Work out the finished part from the listing and answer in its coordinate system (mm). Round coordinates to 2 decimals unless told otherwise and drop trailing zeros. Loops run counter-clockwise (first coordinate to the right, second up) from the corner with the lowest first, then second, coordinate; pieces in that order, holes last.
```python
from build123d import *

# Parameters (mm, degrees)
SKETCH1_R                                         = 82.55
BASE_DEPTH                                        = 6.35
CSK_FOR_6_FLAT_HEAD_MACHINE_SCREW_100_D           = 3.7973
CSK_FOR_6_FLAT_HEAD_MACHINE_SCREW_100_CSINK_D     = 7.0866
CSK_FOR_6_FLAT_HEAD_MACHINE_SCREW_100_CSINK_ANGLE = 100
CUT_EXTRUDE1_DEPTH                                = 117.915899261
F_10_0_1935_DIAMETER_HOLE1_AT_2_COUNT             = 2
F_10_0_1935_DIAMETER_HOLE1_AT_2_PITCH             = 19.05
F_10_0_1935_DIAMETER_HOLE1_AT_3_COUNT             = 2
F_10_0_1935_DIAMETER_HOLE1_AT_3_PITCH             = 25.208780216
F_10_0_1935_DIAMETER_HOLE1_AT_4_COUNT             = 2
F_10_0_1935_DIAMETER_HOLE1_AT_4_PITCH             = 16.51
CIRPATTERN1_COUNT                                 = 3
CUT_EXTRUDE3_DEPTH                                = 117.915899261
FILLET1_R                                         = 7.62
F_8_0_199_DIAMETER_HOLE1_D                        = 5.0546


with BuildPart() as part:
    # Sketch1 → Base (new body)
    with BuildSketch(Plane.XY):
        Circle(SKETCH1_R)
    extrude(amount=BASE_DEPTH)

    # CSK for _6 Flat Head Machine Screw _100 (through all)
    with Locations(Plane(origin=(0, 0, 0), x_dir=(-1, 0, 0), z_dir=(0, 0, -1))):
        with Locations((-41.5, 9), (-41.5, -9), (42.95, 9), (42.95, -9)):
            CounterSinkHole(CSK_FOR_6_FLAT_HEAD_MACHINE_SCREW_100_D / 2, CSK_FOR_6_FLAT_HEAD_MACHINE_SCREW_100_CSINK_D / 2, counter_sink_angle=CSK_FOR_6_FLAT_HEAD_MACHINE_SCREW_100_CSINK_ANGLE)

    # Sketch8 → Cut-Extrude1 (cut, through all)
    with BuildSketch(Plane(origin=(0, 0, 0), x_dir=(-1, 0, 0), z_dir=(0, 0, -1))):
        with BuildLine():
            Line((40, -72.21151224), (-40, -72.21151224))
            ThreePointArc((-40, -72.21151224), (0, -82.55), (40, -72.21151224))
        make_face()
    extrude(amount=-CUT_EXTRUDE1_DEPTH, mode=Mode.SUBTRACT)

    # Sketch12 → #10 (0.1935) Diameter Hole1 (revolve, cut)
    with BuildSketch(Plane(origin=(-40.881368906, -34.601391971, 0), x_dir=(0, 1, 0), z_dir=(1, 0, 0))):
        Polygon((0, 0), (0, 7.826584928), (2.45745, 6.35), (2.45745, 0), align=None)
    f_10_0_1935_diameter_hole1 = revolve(axis=Axis((-40.881368906, -34.601391971, -6.35), (0, 0, 1)), mode=Mode.SUBTRACT)

    # #10 (0.1935) Diameter Hole1 at 2: #10 (0.1935) Diameter Hole1 ×2
    with Locations(*[Vector(-0.4999999999999995, 0.866025403784439, 0) * (i * F_10_0_1935_DIAMETER_HOLE1_AT_2_PITCH) for i in range(1, F_10_0_1935_DIAMETER_HOLE1_AT_2_COUNT)]):
        add(f_10_0_1935_diameter_hole1, mode=Mode.SUBTRACT)

    # #10 (0.1935) Diameter Hole1 at 3: #10 (0.1935) Diameter Hole1 ×2
    with Locations(*[Vector(-0.9450310253789799, 0.32698067384962365, 0) * (i * F_10_0_1935_DIAMETER_HOLE1_AT_3_PITCH) for i in range(1, F_10_0_1935_DIAMETER_HOLE1_AT_3_COUNT)]):
        add(f_10_0_1935_diameter_hole1, mode=Mode.SUBTRACT)

    # #10 (0.1935) Diameter Hole1 at 4: #10 (0.1935) Diameter Hole1 ×2
    with Locations(*[Vector(-0.8660254037844388, -0.49999999999999967, 0) * (i * F_10_0_1935_DIAMETER_HOLE1_AT_4_PITCH) for i in range(1, F_10_0_1935_DIAMETER_HOLE1_AT_4_COUNT)]):
        add(f_10_0_1935_diameter_hole1, mode=Mode.SUBTRACT)

    # CirPattern1: #10 (0.1935) Diameter Hole1 ×3 about axis
    cirpattern1_axis = Axis((0, 0, 0), (0, 0, 1))
    for i in range(1, CIRPATTERN1_COUNT):
        add(f_10_0_1935_diameter_hole1.rotate(cirpattern1_axis, i * 360 / CIRPATTERN1_COUNT), mode=Mode.SUBTRACT)

    # CirPattern1 copy 1 sketch → CirPattern1 copy 1 (revolve, cut)
    with BuildSketch(Plane(origin=(40.881368906, -34.601391971, 0), x_dir=(-0.8660254037844387, -0.4999999999999998, 0), z_dir=(-0.4999999999999998, 0.8660254037844387, 0))):
        Polygon((0, 0), (0, 7.826584928), (2.45745, 6.35), (2.45745, 0), align=None)
    revolve(axis=Axis((40.881368906, -34.601391971, -6.35), (0, 0, 1)), mode=Mode.SUBTRACT)

    # CirPattern1 copy 2 sketch → CirPattern1 copy 2 (revolve, cut)
    with BuildSketch(Plane(origin=(9.525, 52.705, 0), x_dir=(0.8660254037844384, -0.5000000000000004, 0), z_dir=(-0.5000000000000004, -0.8660254037844384, 0))):
        Polygon((0, 0), (0, 7.826584928), (2.45745, 6.35), (2.45745, 0), align=None)
    revolve(axis=Axis((9.525, 52.705, -6.35), (0, 0, 1)), mode=Mode.SUBTRACT)

    # CirPattern1 copy 3 sketch → CirPattern1 copy 3 (revolve, cut)
    with BuildSketch(Plane(origin=(55.179448323, -42.856391971, 0), x_dir=(-0.8660254037844387, -0.4999999999999998, 0), z_dir=(-0.4999999999999998, 0.8660254037844387, 0))):
        Polygon((0, 0), (0, 7.826584928), (2.45745, 6.35), (2.45745, 0), align=None)
    revolve(axis=Axis((55.179448323, -42.856391971, -6.35), (0, 0, 1)), mode=Mode.SUBTRACT)

    # CirPattern1 copy 4 sketch → CirPattern1 copy 4 (revolve, cut)
    with BuildSketch(Plane(origin=(9.525, 69.215, 0), x_dir=(0.8660254037844384, -0.5000000000000004, 0), z_dir=(-0.5000000000000004, -0.8660254037844384, 0))):
        Polygon((0, 0), (0, 7.826584928), (2.45745, 6.35), (2.45745, 0), align=None)
    revolve(axis=Axis((9.525, 69.215, -6.35), (0, 0, 1)), mode=Mode.SUBTRACT)

    # CirPattern1 copy 5 sketch → CirPattern1 copy 5 (revolve, cut)
    with BuildSketch(Plane(origin=(64.704448323, -26.358608029, 0), x_dir=(-0.8660254037844387, -0.4999999999999998, 0), z_dir=(-0.4999999999999998, 0.8660254037844387, 0))):
        Polygon((0, 0), (0, 7.826584928), (2.45745, 6.35), (2.45745, 0), align=None)
    revolve(axis=Axis((64.704448323, -26.358608029, -6.35), (0, 0, 1)), mode=Mode.SUBTRACT)

    # CirPattern1 copy 6 sketch → CirPattern1 copy 6 (revolve, cut)
    with BuildSketch(Plane(origin=(-9.525, 69.215, 0), x_dir=(0.8660254037844384, -0.5000000000000004, 0), z_dir=(-0.5000000000000004, -0.8660254037844384, 0))):
        Polygon((0, 0), (0, 7.826584928), (2.45745, 6.35), (2.45745, 0), align=None)
    revolve(axis=Axis((-9.525, 69.215, -6.35), (0, 0, 1)), mode=Mode.SUBTRACT)

    # Sketch14 → Cut-Extrude3 (cut, through all)
    with BuildSketch(Plane.XY.offset(6.35)):
        with BuildLine():
            Line((-28.575, 28.05), (-123.194399556, 28.05))
            Line((-123.194399556, 28.05), (-123.194399556, 124.921419199))
            Line((-123.194399556, 124.921419199), (-18.415, 124.921419199))
            Line((-18.415, 124.921419199), (-18.415, 38.21))
            ThreePointArc((-18.415, 38.21), (-21.390795103, 31.025795103), (-28.575, 28.05))
        make_face()
        with BuildLine():
            Line((123.194399556, 28.05), (123.194399556, 124.921419199))
            Line((123.194399556, 124.921419199), (18.415, 124.921419199))
            Line((18.415, 124.921419199), (18.415, 38.21))
            ThreePointArc((18.415, 38.21), (21.390795103, 31.025795103), (28.575, 28.05))
            Line((28.575, 28.05), (123.194399556, 28.05))
        make_face()
    extrude(amount=-CUT_EXTRUDE3_DEPTH, mode=Mode.SUBTRACT)

    # Fillet1
    fillet1_edges = [part.edges().sort_by_distance(p)[0] for p in [
        (-18.415, 80.469809711, 3.175),
        (-77.638263762, 28.05, 3.175),
        (18.415, 80.469809711, 3.175),
        (77.638263762, 28.05, 3.175),
    ]]
    fillet(fillet1_edges, radius=FILLET1_R)

    # #8 (0.199) Diameter Hole1 (through all)
    with Locations(Plane(origin=(0, 0, 0), x_dir=(-1, 0, 0), z_dir=(0, 0, -1))):
        with Locations((47.715, -48.08151224), (0.725, -48.08151224), (-46.265, -48.08151224)):
            Hole(F_8_0_199_DIAMETER_HOLE1_D / 2)


solid = part.part
```
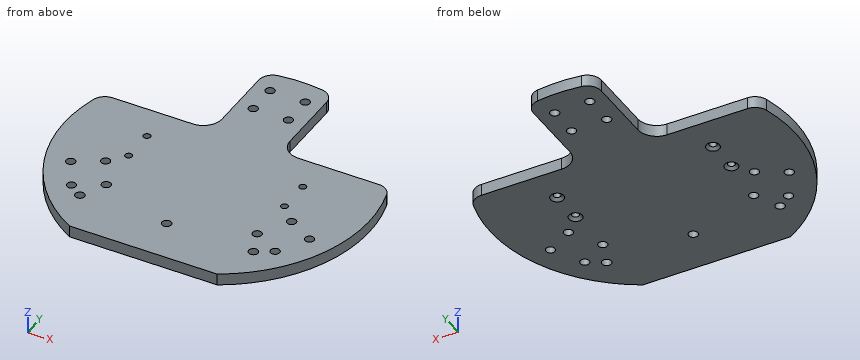
1. Given pin 1 (1 mm diameter, centred on x = 33, y = 15, fed in from -Z); pin 2 (1.5 mm diameter, centred on x = -60.5, z = 1, fed in from -Y); pin 3 (2 mm diameter, centred on y = 7, z = 3, fed in from -X); pin 4 (1.5 mm diameter, centred on x = 26.5, z = 2.5, fed in from +Y), each flat-ended and moving along its own axis, determine where each tip first touches the part or whether it passes through.
Answer key:
pin 1: stops at z = 0
pin 2: stops at y = -56.96
pin 3: stops at x = -82.33
pin 4: stops at y = 28.45
2. Find section A-A (z = 5). Give the number of separate pieces and of enclosed holes in the cut face, then the cut area to 3 significant figures.
Answer key:
separate pieces: 1
enclosed holes: 19
area: 16,400 mm2
3. Consider probe 1 along Y at (x, z) = (41.5, 4.6); probe 2 along X at (y, z) = (-41, 1.5); probe 3 along X at (y, z) = (-9, 4.5). Determine where each line is inside the solid, lowest interval first.
Answer key:
probe 1: y = -71.36 to -36.98, -32.22 to -10.9, -7.1 to 7.1, 10.9 to 28.05
probe 2: x = -71.65 to -56.79, -53.57 to 53.57, 56.79 to 71.65
probe 3: x = -82.06 to -44.85, -41.05 to 39.6, 43.4 to 82.06
4. Find section B-B (y = 9). Write down the section's boundary in (x, z).
Answer key:
outline: (-82.06, 0) - (-46.49, 0) - (-44.85, 1.38) - (-44.85, 6.35) - (-82.06, 6.35) - close; (-41.05, 1.38) - (-39.41, 0) - (37.96, 0) - (39.6, 1.38) - (39.6, 6.35) - (-41.05, 6.35) - close; (43.4, 1.38) - (45.04, 0) - (82.06, 0) - (82.06, 6.35) - (43.4, 6.35) - close
